Source: CAD feature listing. Evaluate the final solid. Frame: model axes, mm. A direction names the side the tool comes from. Round coordinates to 2 decimals unless told otherwise and drop trailing zeros. Loops run counter-clockwise (first coordinate to the right, second up) from the corner with the lowest first, then second, coordinate; pieces in that order, holes last. Notation, with made-up numbers: M -13.75,-28.5 L 15.25,-28.5 A17 cw 15.25,-23.5 Z; hole C -20,15 d7. An arc over 180 degrees is marked long. Answer as a JSON object with one key per item and string values.
from build123d import *

# Parameters (mm, degrees)
F0_R     = 15.875
F0_R_2   = 41.275
F1_DEPTH = 9.525
F0_R_3   = 25.4
F2_DEPTH = 19.05
F3_DEPTH = 19.05
F4_DEPTH = 19.05


with BuildPart() as f1:
    # F0 (on Top) → F1 (new body, symmetric)
    with BuildSketch(Plane.XY):
        with BuildLine():
            ThreePointArc((-28.4345366302, 155.2297973728), (-1.4166406822, 123.860137475), (28.5749999751, 152.4000000228))
            ThreePointArc((28.5749999751, 152.4000000228), (28.5621057669, 153.2583343061), (28.5234347788, 154.1158939584))
            ThreePointArc((28.5234347788, 154.1158939584), (0.5587225598, 180.9695371922), (-28.4345366302, 155.2297973728))
        make_face()
        with Locations((-2.49e-08, 152.4000000228)):
            Circle(F0_R, mode=Mode.SUBTRACT)
        with BuildLine():
            ThreePointArc((28.5234347788, 154.1158939584), (28.5621057669, 153.2583343061), (28.5749999751, 152.4000000228))
            ThreePointArc((28.5749999751, 152.4000000228), (-1.4166406822, 123.860137475), (-28.4345366302, 155.2297973728))
            Line((-28.4345366302, 155.2297973728), (-38.7298241401, 51.7800823041))
            ThreePointArc((-38.7298241401, 51.7800823041), (-44.114260266, 38.4992634308), (-55.8304596742, 30.2468108398))
            Line((-55.8304596742, 30.2468108398), (-226.9598003085, -27.9227065693))
            ThreePointArc((-226.9598003085, -27.9227065693), (-203.4092582541, -33.9896178831), (-193.0604315885, -55.9972808801))
            ThreePointArc((-193.0604315885, -55.9972808801), (-199.8420995066, -74.4791991184), (-216.9681342495, -84.1885376905))
            Line((-216.9681342495, -84.1885376905), (7.0608757552, -47.0986693928))
            Line((7.0608757552, -47.0986693928), (8.4949702479, -46.8612431065))
            ThreePointArc((8.4949702479, -46.8612431065), (38.4017712026, -28.1681485637), (47.2490373051, 5.9723612369))
            Line((47.2490373051, 5.9723612369), (28.5234347788, 154.1158939584))
        make_face()
        Circle(F0_R_2, mode=Mode.SUBTRACT)
        with BuildLine():
            ThreePointArc((7.0608757552, -47.0986693928), (7.7788288983, -46.9854280173), (8.4949702479, -46.8612431065))
            Line((8.4949702479, -46.8612431065), (7.0608757552, -47.0986693928))
        make_face()
        with BuildLine():
            Line((-234.5231416734, -30.4936036204), (-226.9598003085, -27.9227065693))
            ThreePointArc((-226.9598003085, -27.9227065693), (-230.8317532179, -28.9425531326), (-234.5231416734, -30.4936036204))
        make_face()
        with BuildLine():
            ThreePointArc((-193.0604315885, -55.9972808801), (-203.4092582541, -33.9896178831), (-226.9598003085, -27.9227065693))
            Line((-226.9598003085, -27.9227065693), (-234.5231416734, -30.4936036204))
            ThreePointArc((-234.5231416734, -30.4936036204), (-248.7957018858, -64.8770524072), (-216.9681342495, -84.1885376905))
            ThreePointArc((-216.9681342495, -84.1885376905), (-199.8420995066, -74.4791991184), (-193.0604315885, -55.9972808801))
        make_face()
        with Locations((-221.6354315885, -55.9972808801)):
            Circle(F0_R, mode=Mode.SUBTRACT)
    extrude(amount=F1_DEPTH, both=True)

    # F0 (on Top) → F2 (join, symmetric)
    with BuildSketch(Plane.XY):
        with BuildLine():
            ThreePointArc((-193.0604315885, -55.9972808801), (-203.4092582541, -33.9896178831), (-226.9598003085, -27.9227065693))
            Line((-226.9598003085, -27.9227065693), (-234.5231416734, -30.4936036204))
            ThreePointArc((-234.5231416734, -30.4936036204), (-248.7957018858, -64.8770524072), (-216.9681342495, -84.1885376905))
            ThreePointArc((-216.9681342495, -84.1885376905), (-199.8420995066, -74.4791991184), (-193.0604315885, -55.9972808801))
        make_face()
        with Locations((-221.6354315885, -55.9972808801)):
            Circle(F0_R, mode=Mode.SUBTRACT)
        with BuildLine():
            ThreePointArc((-28.4345366302, 155.2297973728), (-1.4166406822, 123.860137475), (28.5749999751, 152.4000000228))
            ThreePointArc((28.5749999751, 152.4000000228), (28.5621057669, 153.2583343061), (28.5234347788, 154.1158939584))
            ThreePointArc((28.5234347788, 154.1158939584), (0.5587225598, 180.9695371922), (-28.4345366302, 155.2297973728))
        make_face()
        with Locations((-2.49e-08, 152.4000000228)):
            Circle(F0_R, mode=Mode.SUBTRACT)
        Circle(F0_R_2)
        Circle(F0_R_3, mode=Mode.SUBTRACT)
    extrude(amount=F2_DEPTH, both=True)

    # F3 (add): a face of the model
    f3_faces = [f1.faces().sort_by_distance(p)[0] for p in [
        (-40.1075667043, 0, 19.05),
    ]]
    extrude(f3_faces, amount=F3_DEPTH)

    # F4 (add): a face of the model
    f4_faces = [f1.faces().sort_by_distance(p)[0] for p in [
        (-40.1075667043, 0, -19.05),
    ]]
    extrude(f4_faces, amount=F4_DEPTH)


solid = f1.part
Item 1: Section A-A on z = 14.5. Return the cut outline in (x, y) (3 decimals), then the cut area to 3 significant figures.
Answer sheet:
{"outline": "M -234.523,-30.494 A28.575 ccw long -226.96,-27.923 Z; C 0,0 d82.55; C 0,152.4 d57.15; hole C -221.635,-55.997 d31.75; hole C 0,0 d50.8; hole C 0,152.4 d31.75", "area": "6,870 mm²"}
Item 2: Section B-B on y = 0. Return the cut outline in (x, z) (3 decimals).
Answer sheet:
{"outline": "M -144.814,-9.525 L -41.275,-9.525 L -41.275,-38.1 L -25.4,-38.1 L -25.4,38.1 L -41.275,38.1 L -41.275,9.525 L -144.814,9.525 Z; M 25.4,-38.1 L 41.275,-38.1 L 41.275,-9.525 L 47.625,-9.525 L 47.625,9.525 L 41.275,9.525 L 41.275,38.1 L 25.4,38.1 Z"}
Item 3: Line query: probe 1 along Y at (x, z) = (0, -7) (3 decimals); probe 2 along Z at (x, y) = (-93.5, -60) (3 decimals); probe 3 along Y at (x, z) = (-13, 27). Output: solid intervals per line, ascending. Write a range as from..to.
Answer sheet:
{"probe 1": "y = -48.268..-25.4, 25.4..136.525, 168.275..180.975", "probe 2": "z = -9.525..9.525", "probe 3": "y = -39.17..-21.82, 21.82..39.17"}
Item 4: Contact query for flat-ended pins moving along their axis: pin 1 Ø3 at (x, y) = (-230.5, -29) entering from -Z; pin 2 Ø1 at (x, y) = (-32, 65.5) entering from -Z (3 decimals); pin 3 Ø12 at (y, z) = (62.5, 6.5) entering from +X. Output: stop coordinate, or through.
Answer sheet:
{"pin 1": "stops at z = -19.05", "pin 2": "stops at z = -9.525", "pin 3": "stops at x = 40.86"}
Item 5: Pull-direction query (X, two-part tool) for faces 6 (the flat face through (-209, -68, -19.05)), 7 (the cylindrical face through (-5.506, -24.796, -0.533)), 8 (the flat face through (-230.69, -29.19, -14.22)); classes: pulls with the +X half, pulls with the -X half, needs draft (parallel to the pull), parting line crosses it, or undercut.
Answer sheet:
{"face 6": "needs draft", "face 7": "undercut", "face 8": "pulls with the -X half"}
Item 6: Access query for faces 1 (the flat face through (-230.69, -29.19, 14.22)), 2 (the flat face through (12, 140, 19.05)), 3 (the flat face through (-60, 1, 9.525)), 4 (the flat face through (-60, 1, -9.525)), 5 (the flat face through (12, 140, -19.05)). Directions: +Z, -Z, +X, -X, +Y, -Y. A direction counts if a zero-diameter tool reaches every point of the face in a straight line with its end or side. Return the directions, or none.
Answer sheet:
{"face 1": "+Z, -X, +Y", "face 2": "+Z, +X, -X, +Y", "face 3": "+Z", "face 4": "-Z", "face 5": "-Z, +X, -X, +Y"}
Item 7: Section C-C on x = 0. Return the cut outline in (y, z) (3 decimals).
Answer sheet:
{"outline": "M -48.268,-9.525 L -41.275,-9.525 L -41.275,-38.1 L -25.4,-38.1 L -25.4,38.1 L -41.275,38.1 L -41.275,9.525 L -48.268,9.525 Z; M 25.4,-38.1 L 41.275,-38.1 L 41.275,-9.525 L 123.825,-9.525 L 123.825,-19.05 L 136.525,-19.05 L 136.525,19.05 L 123.825,19.05 L 123.825,9.525 L 41.275,9.525 L 41.275,38.1 L 25.4,38.1 Z; M 168.275,-19.05 L 180.975,-19.05 L 180.975,19.05 L 168.275,19.05 Z"}
Item 8: Section D-D on z = -30.5. Return the cut outline in (x, y) (3 decimals).
Answer sheet:
{"outline": "C 0,0 d82.55; hole C 0,0 d50.8"}
